Work out the finished part from the listing and answer in its coordinate system (mm). A direction names the side the tool comes from. Coordinates: 2 decimals unless noted, no trailing zeros. Order: outer loops, then holes, each group sorted by start corner. A loop starts at its lowest first (then second) coordinate and runs counter-clockwise, first axis right, second up. Notation, with made-up numbers: (86, 88) -> (126, 88) arc R25 cw to (126, 110) -> close; hole circle Ø6 at (-12.5, 47). An arc over 180 degrees is marked (long way). Use one line per item in the form item = value.
from build123d import *

# Parameters (mm, degrees)
F0_R        = 1.75
F1_DEPTH    = 5
F2_W        = 5
F2_H        = 18.5
F3_DEPTH    = 100
F4_W        = 18.5
F4_H        = 5
F5_DEPTH    = 70.1
F6_R        = 17.5
F6_R_2      = 2
F7_DEPTH    = 25
F8_SIZE     = 3
F9_T1_DEPTH = 19.3723210726


# Not quite as in the source:
# - a fillet or chamfer that OpenCascade refuses, or shapes differently, is made with other operations: its cross-section is extruded or revolved along the edge and cut away or added


with BuildPart() as f1:
    # F0 (on Top) → F1 (new body)
    with BuildSketch(Plane.XY):
        with BuildLine():
            ThreePointArc((-11.1, 0), (0, 11.1), (11.1, 0))
            Line((11.1, 0), (40.05, 0))
            Line((40.05, 0), (40.05, 21.25))
            Line((40.05, 21.25), (-40.05, 21.25))
            Line((-40.05, 21.25), (-40.05, 0))
            Line((-40.05, 0), (-11.1, 0))
        make_face()
        with Locations((-15.5, 15.5)):
            Circle(F0_R, mode=Mode.SUBTRACT)
        with Locations((15.5, 15.5)):
            Circle(F0_R, mode=Mode.SUBTRACT)
    extrude(amount=F1_DEPTH)

    # F2 (on face) → F3 (join)
    with BuildSketch(Plane.XY.offset(5)):
        with Locations((-37.55, 12)):
            Rectangle(F2_W, F2_H)
        with Locations((37.55, 12)):
            Rectangle(F2_W, F2_H)
    extrude(amount=F3_DEPTH)

    # F4 (on face) → F5 (join, through all)
    with BuildSketch(Plane(origin=(35.05, 0, 0), x_dir=(0, -1, 0), z_dir=(-1, 0, 0))):
        with Locations((-12, 55)):
            Rectangle(F4_W, F4_H)
    extrude(amount=F5_DEPTH)

    # F6 (on face) → F7 (cut)
    with BuildSketch(Plane(origin=(0, 0, 52.5), x_dir=(1, 0, 0), z_dir=(0, 0, -1))):
        Circle(F6_R)
        with Locations((-28.55, -8)):
            Circle(F6_R_2)
        with Locations((28.55, -8)):
            Circle(F6_R_2)
    extrude(amount=-F7_DEPTH, mode=Mode.SUBTRACT)

    # F8
    f8_edges = [f1.edges().sort_by_distance(p)[0] for p in [
        (-40.05, 10.625, 0),
        (40.05, 10.625, 0),
        (-40.05, 12, 105),
        (40.05, 12, 105),
    ]]
    chamfer(f8_edges, length=F8_SIZE)

    # F9: chamfer of 3 on 2 edges, made by hand

    # F9_s2 → F9_t1 (cut)
    with BuildSketch(Plane.XY.offset(45.3138394637)):
        with BuildLine():
            Line((-20.1561629778, 2.678911963), (-16.6075492446, 5.288253662))
            Line((-16.6075492446, 5.288253662), (-16.5502776109, 5.270366237))
            ThreePointArc((-16.5502776109, 5.270366237), (-16.9692117334, 4.0248544257), (-17.2233233798, 2.7405714286))
            Line((-17.2233233798, 2.7405714286), (-17.2825779327, 2.69))
            ThreePointArc((-17.2825779327, 2.69), (-18.7193704553, 2.69), (-20.1561629778, 2.618911963))
            Line((-20.1561629778, 2.618911963), (-20.1561629778, 2.678911963))
        make_face()
        with BuildLine():
            Line((20.1561629778, 2.678911963), (16.6075492446, 5.288253662))
            Line((16.6075492446, 5.288253662), (16.5502776109, 5.270366237))
            ThreePointArc((16.5502776109, 5.270366237), (16.9692117334, 4.0248544257), (17.2233233798, 2.7405714286))
            Line((17.2233233798, 2.7405714286), (17.2825779327, 2.69))
            ThreePointArc((17.2825779327, 2.69), (18.7193704553, 2.69), (20.1561629778, 2.618911963))
            Line((20.1561629778, 2.618911963), (20.1561629778, 2.678911963))
        make_face()
    extrude(amount=F9_T1_DEPTH, mode=Mode.SUBTRACT)


solid = f1.part
(1) Section B-B on x = -15.5 is taken. Write down the section's boundary in (y, z).
Data:
outline = (0, 0) -> (13.75, 0) -> (13.75, 5) -> (0, 5) -> close; (8.12, 52.5) -> (21.25, 52.5) -> (21.25, 57.5) -> (8.12, 57.5) -> close; (17.25, 0) -> (21.25, 0) -> (21.25, 5) -> (17.25, 5) -> close
(2) The mould has two halves that part along Y. Classify faces 6 (the cylindrical face through (-26.642, 7.399, 54.965)), 7 (the flat face through (38.57, 11.87, 103.48)), 8 (the flat face through (18.405, 3.966, 54.965)): released by +Y, released by -Y, zero draft, split by the parting line, or undercut.
Data:
face_6 = undercut
face_7 = zero draft
face_8 = released by -Y
(3) Straight lines are drawn through the part: line 1 along X through (y, z) = (13, 23); line 2 along Z through (x, y) = (-32, 18); line 3 along Y through (x, z) = (-15.5, 3.55). For each, find the intervals that lie inside material, in ascending order.
Data:
line_1 = -40.05 to -35.05, 35.05 to 40.05
line_2 = 0 to 5, 52.5 to 57.5
line_3 = 0 to 13.75, 17.25 to 21.25
(4) Section A-A on z = 65.5 is taken. Write down the section's boundary in (x, y), plus the area to 3 significant figures.
Data:
outline = (-40.05, 2.75) -> (-35.05, 2.75) -> (-35.05, 21.25) -> (-40.05, 21.25) -> close; (35.05, 2.75) -> (40.05, 2.75) -> (40.05, 21.25) -> (35.05, 21.25) -> close
area = 185 mm²
(5) Section D-D on x = 0 is taken. Write down the section's boundary in (y, z).
Data:
outline = (11.1, 0) -> (21.25, 0) -> (21.25, 5) -> (11.1, 5) -> close; (17.5, 52.5) -> (21.25, 52.5) -> (21.25, 57.5) -> (17.5, 57.5) -> close
(6) Section C-C on z = 54 is taken. Write down the section's boundary in (x, y).
Data:
outline = (-40.05, 2.75) -> (-20.06, 2.75) -> (-16.7, 5.22) arc R17.5 cw to (16.7, 5.22) -> (20.06, 2.75) -> (40.05, 2.75) -> (40.05, 21.25) -> (-40.05, 21.25) -> close; hole circle Ø4 at (-28.55, 8); hole circle Ø4 at (28.55, 8)
(7) Which of the six approach directions +Z, -Z, +X, -X, +Y, -Y give full straight-line access (tool end or side, diameter ignored) to faces 1 (the flat face through (35.05, 12, 28)), 2 (the cylindrical face through (26.552, 7.912, 54.965)), 3 (the cylindrical face through (15.272, 17.235, 2.465)), 4 (the flat face through (0, 18, 57.5)), 5 (the cylindrical face through (-0.311, 17.497, 54.965))?
Data:
face_1 = +Y, -Y
face_2 = +Z
face_3 = -Z
face_4 = +Z, +Y, -Y
face_5 = +Z, -Y
(8) Each of these flat-tipped pins is pushed along its axis until it touches: P1, Ø5, axis at x = -28.55, y = 8, coming from the +Z side; P2, Ø22, axis at x = 33, z = 50.5, coming from the -Y side; P3, Ø3.5, axis at x = 28.55, y = 8, coming from the +Z side. Where does it stop, or does it pass through?
Data:
P1 = 57.5
P2 = 2.75
P3 = 5
